Source: CAD feature listing. Evaluate the final solid. Frame: model axes, mm. A direction names the side the tool comes from. Give positions to 0.01 mm unless a question says otherwise; leave off trailing zeros. Loops run counter-clockwise (first coordinate to the right, second up) from the corner with the lowest first, then second, coordinate; pieces in that order, holes last. Notation, with made-up numbers: (-35.75, 78) -> (-15.75, 78) arc R7 ccw to (-15.75, 87) -> close; hole circle Ø2 at (3.5, -12). An arc over 180 degrees is marked (long way). Return JSON: item names as keys, results as strings. Group by question number.
(1) Draft query along Z for faces 3 (the face through (-17, 0, -30)), 4 (the face through (1, -10, 1)). Return one class per face: released by +Z, released by -Z, zero draft, split by the parting line, or undercut.
(2) Cut plane B-B on y = 28. Give the number of separate pieces and of enclosed holes in the cut face, then the cut area to 3 significant figures.
(3) Access query for faces 1 (the face through (-30, 75, 47)), 2 (the face through (1, 0, 1)). Directions: +Z, -Z, +X, -X, +Y, -Y. A direction counts if a zero-diameter tool reaches every point of the face in a straight line with its end or side. Return the directions, or none.
(4) Cut plane C-C on z = 0. Return loops of the section in (x, y).
(5) Pin query (flat end, axial travel): pin 1 (23 mm diameter, centred on x = 19, z = -27.5, fed in from +Y); pin 2 (8 mm diameter, centred on y = 12, z = -29, fed in from +X); pin 3 (8 mm diameter, centred on y = 34, z = 5, fed in from -X). Return the tip coordinate at first contact, or that it passes through.
(6) Cut plane A-A on x = 0. Return loops of the section in (y, z), then the cut area to 3 significant figures.
(7) Ray query, line 1 (X direction, y = 48, z = 0); line 2 (Z direction, x = 40.5, y = 12); line 3 (X direction, y = 47, z = 30). Return the intervals inside material, ascending. Write a range as from..to.
(8) Cut plane D-D on y = -1.5. Return loops of the section in (x, z), then the cut area to 3 significant figures.
```python
from build123d import *

# Parameters (mm, degrees)
SKETCH2_R             = 15
SKETCH2_R_2           = 10.5
BOSS_EXTRUDE1_DEPTH   = 75
BOSS_EXTRUDE1_2_DEPTH = 75
BOSS_EXTRUDE1_3_DEPTH = 75
BOSS_EXTRUDE1_4_DEPTH = 75
BOSS_EXTRUDE1_5_DEPTH = 75
BOSS_EXTRUDE1_6_DEPTH = 75
SKETCH2_R_3           = 57.5
SKETCH2_R_4           = 55
BOSS_EXTRUDE1_7_DEPTH = 75
SKETCH3_R             = 57.5
BOSS_EXTRUDE2_DEPTH   = 10
CHAMFER2_SIZE         = 5
CHAMFER2_SIZE_2       = 8.660254038
FILLET1_R             = 5


with BuildPart() as part:
    # Sketch2 → Boss-Extrude1 (new body)
    with BuildSketch(Plane(origin=(0, 0, 0), x_dir=(1, 0, 0), z_dir=(0, 1, 0))):
        with Locations(Location((-34.641016151, 0, 0), (0, 0, 270))):
            Circle(SKETCH2_R)
        with Locations(Location((-34.641016151, 0, 0), (0, 0, 270))):
            Circle(SKETCH2_R_2, mode=Mode.SUBTRACT)
    extrude(amount=BOSS_EXTRUDE1_DEPTH)



with BuildPart() as body_2:
    # Sketch2 → Boss-Extrude1 2 (new body)
    with BuildSketch(Plane(origin=(0, 0, 0), x_dir=(1, 0, 0), z_dir=(0, 1, 0))):
        with Locations(Location((-17.320508076, 30, 0), (0, 0, 270))):
            Circle(SKETCH2_R)
        with Locations(Location((-17.320508076, 30, 0), (0, 0, 270))):
            Circle(SKETCH2_R_2, mode=Mode.SUBTRACT)
    extrude(amount=BOSS_EXTRUDE1_2_DEPTH)


with BuildPart() as body_3:
    # Sketch2 → Boss-Extrude1 3 (new body)
    with BuildSketch(Plane(origin=(0, 0, 0), x_dir=(1, 0, 0), z_dir=(0, 1, 0))):
        with Locations(Location((17.320508076, 30, 0), (0, 0, 270))):
            Circle(SKETCH2_R)
        with Locations(Location((17.320508076, 30, 0), (0, 0, 270))):
            Circle(SKETCH2_R_2, mode=Mode.SUBTRACT)
    extrude(amount=BOSS_EXTRUDE1_3_DEPTH)


with BuildPart() as body_4:
    # Sketch2 → Boss-Extrude1 4 (new body)
    with BuildSketch(Plane(origin=(0, 0, 0), x_dir=(1, 0, 0), z_dir=(0, 1, 0))):
        with Locations(Location((34.641016151, 0, 0), (0, 0, 270))):
            Circle(SKETCH2_R)
        with Locations(Location((34.641016151, 0, 0), (0, 0, 270))):
            Circle(SKETCH2_R_2, mode=Mode.SUBTRACT)
    extrude(amount=BOSS_EXTRUDE1_4_DEPTH)


with BuildPart() as body_5:
    # Sketch2 → Boss-Extrude1 5 (new body)
    with BuildSketch(Plane(origin=(0, 0, 0), x_dir=(1, 0, 0), z_dir=(0, 1, 0))):
        with Locations(Location((17.320508076, -30, 0), (0, 0, 270))):
            Circle(SKETCH2_R)
        with Locations(Location((17.320508076, -30, 0), (0, 0, 270))):
            Circle(SKETCH2_R_2, mode=Mode.SUBTRACT)
    extrude(amount=BOSS_EXTRUDE1_5_DEPTH)


with BuildPart() as body_6:
    # Sketch2 → Boss-Extrude1 6 (new body)
    with BuildSketch(Plane(origin=(0, 0, 0), x_dir=(1, 0, 0), z_dir=(0, 1, 0))):
        with Locations(Location((-17.320508076, -30, 0), (0, 0, 270))):
            Circle(SKETCH2_R)
        with Locations(Location((-17.320508076, -30, 0), (0, 0, 270))):
            Circle(SKETCH2_R_2, mode=Mode.SUBTRACT)
    extrude(amount=BOSS_EXTRUDE1_6_DEPTH)


with BuildPart() as body_7:
    # Sketch2 → Boss-Extrude1 7 (new body)
    with BuildSketch(Plane(origin=(0, 0, 0), x_dir=(1, 0, 0), z_dir=(0, 1, 0))):
        with Locations(Location((0, 0, 0), (0, 0, 270))):
            Circle(SKETCH2_R_3)
        with Locations(Location((0, 0, 0), (0, 0, 270))):
            Circle(SKETCH2_R_4, mode=Mode.SUBTRACT)
    extrude(amount=BOSS_EXTRUDE1_7_DEPTH)


with BuildPart() as part_1:
    add(part.part)

    add(body_2.part)  # Boss-Extrude2 merges body 2

    add(body_3.part)  # Boss-Extrude2 merges body 3

    add(body_4.part)  # Boss-Extrude2 merges body 4

    add(body_5.part)  # Boss-Extrude2 merges body 5

    add(body_6.part)  # Boss-Extrude2 merges body 6

    add(body_7.part)  # Boss-Extrude2 merges body 7
    # Sketch3 → Boss-Extrude2 (add)
    with BuildSketch(Plane.XZ):
        with Locations(Location((0, 0, 0), (0, 0, 270))):
            Circle(SKETCH3_R)
    extrude(amount=BOSS_EXTRUDE2_DEPTH)

    # Chamfer2
    # the kernel refuses this chamfer: 8.660254038, 5 mm, written as the material it takes off along each edge
    with BuildSketch(Plane(origin=(-17.320508076, 75, -30), x_dir=(0, 0, 1), z_dir=(-1, 0, 0))) as chamfer2_piece_1:
        Polygon((10.5 + CHAMFER2_SIZE, 0), (10.5, -CHAMFER2_SIZE_2), (10.5, 0), align=None)
    revolve(axis=Axis((-17.320508076, 75, -30), (0, 1, 0)), mode=Mode.SUBTRACT)
    with BuildSketch(Plane(origin=(-34.641016151, 75, 0), x_dir=(0, 0, 1), z_dir=(-1, 0, 0))) as chamfer2_piece_2:
        Polygon((10.5 + CHAMFER2_SIZE, 0), (10.5, -CHAMFER2_SIZE_2), (10.5, 0), align=None)
    revolve(axis=Axis((-34.641016151, 75, 0), (0, 1, 0)), mode=Mode.SUBTRACT)
    with BuildSketch(Plane(origin=(-17.320508076, 75, 30), x_dir=(0, 0, 1), z_dir=(-1, 0, 0))) as chamfer2_piece_3:
        Polygon((10.5 + CHAMFER2_SIZE, 0), (10.5, -CHAMFER2_SIZE_2), (10.5, 0), align=None)
    revolve(axis=Axis((-17.320508076, 75, 30), (0, 1, 0)), mode=Mode.SUBTRACT)
    with BuildSketch(Plane(origin=(17.320508076, 75, 30), x_dir=(0, 0, 1), z_dir=(-1, 0, 0))) as chamfer2_piece_4:
        Polygon((10.5 + CHAMFER2_SIZE, 0), (10.5, -CHAMFER2_SIZE_2), (10.5, 0), align=None)
    revolve(axis=Axis((17.320508076, 75, 30), (0, 1, 0)), mode=Mode.SUBTRACT)
    with BuildSketch(Plane(origin=(34.641016151, 75, 0), x_dir=(0, 0, 1), z_dir=(-1, 0, 0))) as chamfer2_piece_5:
        Polygon((10.5 + CHAMFER2_SIZE, 0), (10.5, -CHAMFER2_SIZE_2), (10.5, 0), align=None)
    revolve(axis=Axis((34.641016151, 75, 0), (0, 1, 0)), mode=Mode.SUBTRACT)
    with BuildSketch(Plane(origin=(17.320508076, 75, -30), x_dir=(0, 0, 1), z_dir=(-1, 0, 0))) as chamfer2_piece_6:
        Polygon((10.5 + CHAMFER2_SIZE, 0), (10.5, -CHAMFER2_SIZE_2), (10.5, 0), align=None)
    revolve(axis=Axis((17.320508076, 75, -30), (0, 1, 0)), mode=Mode.SUBTRACT)

    # Fillet1
    fillet1_edges = [part_1.edges().sort_by_distance(p)[0] for p in [
        (0, -10, 57.5),
    ]]
    fillet(fillet1_edges, radius=FILLET1_R)


solid = part_1.part
```
Answers:
{
 "1": {"face 3": "undercut", "face 4": "zero draft"},
 "2": {"separate pieces": "7", "enclosed holes": "7", "area": "3,050 mm²"},
 "3": {"face 1": "+Z, -Z, +X, -X, +Y", "face 2": "+Y"},
 "4": {"outline": "(-57.5, -5) arc R5 ccw to (-52.5, -10) -> (52.5, -10) arc R5 ccw to (57.5, -5) -> (57.5, 75) -> (55, 75) -> (55, 0) -> (49.64, 0) -> (49.64, 74.13) -> (45.14, 66.34) -> (45.14, 0) -> (24.14, 0) -> (24.14, 66.34) -> (19.64, 74.13) -> (19.64, 0) -> (-19.64, 0) -> (-19.64, 74.13) -> (-24.14, 66.34) -> (-24.14, 0) -> (-45.14, 0) -> (-45.14, 66.34) -> (-49.64, 74.13) -> (-49.64, 0) -> (-55, 0) -> (-55, 75) -> (-57.5, 75) -> close"},
 "5": {"pin 1": "y = 73.29", "pin 2": "x = 51.78", "pin 3": "x = -57.49"},
 "6": {"outline": "(-10, -52.5) arc R5 ccw to (-5, -57.5) -> (75, -57.5) -> (75, -55) -> (0, -55) -> (0, 55) -> (75, 55) -> (75, 57.5) -> (-5, 57.5) arc R5 ccw to (-10, 52.5) -> close", "area": "1,510 mm²"},
 "7": {"line 1": "-57.5..-55, -49.64..-45.14, -24.14..-19.64, 19.64..24.14, 45.14..49.64, 55..57.5", "line 2": "-40.82..-37.21, -13.81..-8.71, 8.71..13.81, 37.21..40.82", "line 3": "-49.05..-46.1, -32.32..-27.82, -6.82..-2.32, 2.32..6.82, 27.82..32.32, 46.1..49.05"},
 "8": {"outline": "circle Ø115 at (0, 0)", "area": "10,400 mm²"}
}
